```python
from build123d import *

# Parameters (mm, degrees)
SKETCH_W        = 88.694274
SKETCH_H        = 25.15924
PAD_DEPTH       = 3
FILLET_R        = 12
POCKET_DEPTH    = 5
SKETCH002_W     = 6.815415
SKETCH002_H     = 25.06178
PAD001_DEPTH    = 22
FILLET001_R     = 3
SKETCH003_W     = 6.847126
SKETCH003_H     = 18.152864
POCKET001_DEPTH = 25.11151
SKETCH004_R     = 1.351161
POCKET002_DEPTH = 14
SKETCH005_W     = 22.611487
SKETCH005_H     = 24.415462
PAD002_DEPTH    = 29
FILLET002_R     = 11
PAD003_DEPTH    = 5
SKETCH007_R     = 2.367202
POCKET003_DEPTH = 17.788351
SKETCH008_R     = 5.409327
POCKET004_DEPTH = 24.788351


with BuildPart() as part:
    # Sketch → Pad (new body)
    with BuildSketch(Plane.XY):
        Rectangle(SKETCH_W, SKETCH_H)
    extrude(amount=PAD_DEPTH)

    # Fillet
    fillet_edges = [part.edges().sort_by_distance(p)[0] for p in [
        (44.347137, -12.57962, 1.5),
        (44.347137, 12.57962, 1.5),
    ]]
    fillet(fillet_edges, radius=FILLET_R)

    # Sketch001 (on Face5 of Fillet) → Pocket (cut)
    with BuildSketch(Plane.XY.offset(3)):
        with BuildLine():
            ThreePointArc((18.869435, 3.66242), (15.207015, 0), (18.869435, -3.66242))
            Line((18.869435, -3.66242), (33.519115, -3.66242))
            ThreePointArc((33.519115, -3.66242), (37.181535, 0), (33.519115, 3.66242))
            Line((33.519115, 3.66242), (18.869435, 3.66242))
        make_face()
    extrude(amount=-POCKET_DEPTH, mode=Mode.SUBTRACT)

    # Sketch002 (on Face5 of Pocket) → Pad001 (join)
    with BuildSketch(Plane.XY.offset(3)):
        with Locations((-40.843948, 0)):
            Rectangle(SKETCH002_W, SKETCH002_H)
    extrude(amount=PAD001_DEPTH)

    # Fillet001
    fillet001_edges = [part.edges().sort_by_distance(p)[0] for p in [
        (-40.843949, -12.53089, 25),
        (-40.843948, 12.53089, 25),
    ]]
    fillet(fillet001_edges, radius=FILLET001_R)

    # Sketch003 (on Face2 of Fillet001) → Pocket001 (cut, through all)
    with BuildSketch(Plane.XZ.offset(12.53089)):
        with Locations((-37.261145, 22.292999)):
            Rectangle(SKETCH003_W, SKETCH003_H)
    extrude(amount=-POCKET001_DEPTH, mode=Mode.SUBTRACT)

    # Sketch004 (on Face18 of Pocket001) → Pocket002 (cut)
    with BuildSketch(Plane.YZ.offset(-40.684708)):
        with Locations((-8.64271, 21.337582)):
            Circle(SKETCH004_R)
        with Locations((8.64271, 21.337582)):
            Circle(SKETCH004_R)
    extrude(amount=-POCKET002_DEPTH, mode=Mode.SUBTRACT)

    # Sketch005 (on Face2 of Pocket002) → Pad002 (join)
    with BuildSketch(Plane.XY.offset(3)):
        with Locations((-4.538261, 0)):
            Rectangle(SKETCH005_W, SKETCH005_H)
    extrude(amount=PAD002_DEPTH)

    # Fillet002
    fillet002_edges = [part.edges().sort_by_distance(p)[0] for p in [
        (6.767482, 0, 32),
        (-15.844005, 0, 32),
    ]]
    fillet(fillet002_edges, radius=FILLET002_R)

    # Sketch006 (on Face1 of Fillet002) → Pad003 (join, symmetric)
    with BuildSketch(Plane.XZ.offset(0.207731)):
        with BuildLine():
            ThreePointArc((-10.734413, 19.926899), (-9.362729, 11.672937), (-1.108767, 13.044622))
            Line((-1.108767, 13.044622), (10.583898, 29.398141))
            ThreePointArc((10.583898, 29.398141), (9.212214, 37.652103), (0.958252, 36.280419))
            Line((0.958252, 36.280419), (-10.734413, 19.926899))
        make_face()
    extrude(amount=PAD003_DEPTH, both=True)

    # Sketch007 (on Face11 of Pad003) → Pocket003 (cut, through all)
    with BuildSketch(Plane.XZ.offset(5.207731)):
        with Locations((5.724531, 33.13562)):
            Circle(SKETCH007_R)
    extrude(amount=-POCKET003_DEPTH, mode=Mode.SUBTRACT)

    # Sketch008 (on Face1 of Pocket003) → Pocket004 (cut, through all)
    with BuildSketch(Plane.XZ.offset(12.207731)):
        with Locations((-4.466556, 21.352194)):
            Circle(SKETCH008_R)
    extrude(amount=-POCKET004_DEPTH, mode=Mode.SUBTRACT)


solid = part.part
```
For this review, take the finished solid that the model builds, in its own axes (mm). A direction names the side the tool comes from. Round coordinates to 2 decimals unless told otherwise and drop trailing zeros. Write each loop counter-clockwise with the first axis right and the second up, starting at its lowest first coordinate (ties: lowest second). Pieces come first, ordered by that corner, then holes. Notation, with made-up numbers: (-28, 21.5) -> (-2, 21.5) arc R9 ccw to (-2, 29.5) -> close; hole circle Ø5 at (2.25, -35). An arc over 180 degrees is marked (long way). One line per question, with ' | ' between items. Start each with the question number.
1) Wall thickness on line 1 along X through (y, z) = (4, 21); line 2 along X through (y, z) = (5.5, 20); line 3 along X through (y, z) = (-2.25, 3.5): over which ranges is each line inside the solid? List them lowest first.
2) Add section B-B (z = 11). Write out the cut boundary in (x, y).
3) Add section D-D (z = 18). Write out the cut boundary in (x, y).
4) Add section A-A (x = 29). Write out the cut boundary in (y, z).
5) For pin 1 Ø0.5 at (x, y) = (-4.5, 4.5) entering from +Z; pin 2 Ø12.5 at (x, y) = (-21, -1.5) entering from +Z; pin 3 Ø5 at (x, z) = (6, 6.5) entering from -Y, all flat-tipped, find the tip position at first contact; note any pin that passes through.
6) Mouldability with a two-part tool opening along Z and no side actions: class faces 4 (the cylindrical face through (-42.443, -11.675, 24.098)), 5 (the cylindrical face through (3.36, -0.28, 33.24)), 6 (the flat face through (26, 3.662, 2)), 7 (the flat face through (-1, 0, 0)) as +Z half, -Z half, draft (parallel to the pull), parting line (faces both ways), or undercut.
7) Add section C-C (y = 11). Write out the cut boundary in (x, z), and give its area (3 significant figures).
8) Machinability: for faces 1 (the cylindrical face through (-42.443, 8.467, 22.677)), 2 (the cylindrical face through (-42.443, 11.675, 24.098)), 3 (the flat face through (-5, -12.208, 14)), which of the approach directions +Z, -Z, +X, -X, +Y, -Y give a long, thin tool a straight path to every point of the face, cutting with its end or side? Answer none if there is none.
Reported:
1) line 1: x = -44.25 to -40.68, -15.84 to -9.86, 0.93 to 6.77 | line 2: x = -44.25 to -40.68, -15.84 to -9.7, 0.77 to 6.77 | line 3: x = -44.25 to -37.44, -15.84 to 6.77
2) outline: (-44.25, -12.53) -> (-37.44, -12.53) -> (-37.44, 12.53) -> (-44.25, 12.53) -> close; (-15.84, -12.21) -> (6.77, -12.21) -> (6.77, 12.21) -> (-15.84, 12.21) -> close
3) outline: (-44.25, -12.53) -> (-40.68, -12.53) -> (-40.68, 12.53) -> (-44.25, 12.53) -> close; (-15.84, -12.21) -> (-8.71, -12.21) -> (-8.71, 12.21) -> (-15.84, 12.21) -> close; (-0.22, -12.21) -> (6.77, -12.21) -> (6.77, 12.21) -> (-0.22, 12.21) -> close
4) outline: (-12.58, 0) -> (-3.66, 0) -> (-3.66, 3) -> (-12.58, 3) -> close; (3.66, 0) -> (12.58, 0) -> (12.58, 3) -> (3.66, 3) -> close
5) pin 1: stops at z = 32 | pin 2: stops at z = 25.78 | pin 3: stops at y = -12.21
6) face 4: +Z half | face 5: undercut | face 6: draft | face 7: -Z half
7) outline: (-44.35, 0) -> (38.3, 0) -> (38.3, 3) -> (6.77, 3) -> (6.77, 21) arc R11 ccw to (-4.23, 32) -> (-4.84, 32) arc R11 ccw to (-15.84, 21) -> (-15.84, 3) -> (-37.44, 3) -> (-37.44, 13.22) -> (-40.68, 13.22) -> (-40.68, 24.62) -> (-44.25, 24.62) -> (-44.25, 3) -> (-44.35, 3) -> close; hole circle Ø10.82 at (-4.47, 21.35) | area: 870 mm²
8) face 1: -X | face 2: +Z, -X, +Y | face 3: +Z, +X, -Y
